Verification items for the finished model (mm, model axes). Face numbers are marked on the shaded views. A direction names the side the tool comes from. Coordinates: 2 decimals unless noted, no trailing zeros. Order: outer loops, then holes, each group sorted by start corner. A loop starts at its lowest first (then second) coordinate and runs counter-clockwise, first axis right, second up.
Q1. Cross-section at A-A, the plane y = 0. Count the separate pieces of the cut face and the enclosed holes in it, and give its area (3 significant figures).
Q2. Set-up check for the marked faces 4 and 5: record each of +Z, -Z, +X, -X, +Y, -Y from which the full face is reachable in a straight line by a thin tool's end or side.
Q3. Thickness scan on line 1 (Y direction, x = -39.5, z = -2); line 2 (X direction, y = 7.5, z = -2.25); line 3 (X direction, y = -6, z = -6). Record the ranges inside material, lowest first.
Q4. Depth check by flat-ended pin: P1, Ø5, axis at x = 1.5, z = -4.5, coming from the +Y side; P2, Ø5, axis at x = -24.18, y = 0, coming from the +Z side; P3, Ø2, axis at x = -18.5, z = -4, coming from the +Y side; P4, Ø3, axis at y = 3.5, z = -6, coming from the +X side. Enter the tip coordinate at first touch or a pass-through.
Q5. Draft check along X on the marked faces 1, 2 and 3. Enter one of: pulls with the +X half, pulls with the -X half, needs draft (parallel to the pull), parting line crosses it, or undercut.
Q6. Cross-section at D-D, the plane x = 55. Record the boundary of the cut face in (y, z).
Q7. Cross-section at B-B, the plane y = 33. Record the boundary of the cut face in (x, z).
from build123d import *

# Parameters (mm, degrees)
SKETCH6_R                        = 29
SKETCH6_R_2                      = 20
INNER_RING_DEPTH                 = 10
MOTOR_CONNECTOR_CUT_DEPTH        = 10
SKETCH8_R                        = 2.25
MOTOR_CONNECTOR_HOLES_DEPTH      = 1
MOTOR_CONNECTOR_HOLES_DEPTH_BACK = 18
MIDDLE_PATTERN_DEPTH             = 10
SKETCH9_R                        = 60
SKETCH9_R_2                      = 50
SKETCH9_R_3                      = 2.5
BOSS_EXTRUDE1_DEPTH              = 10


with BuildPart() as part:
    # Sketch6 → Inner Ring (new body)
    with BuildSketch(Plane.XY):
        Circle(SKETCH6_R)
        Circle(SKETCH6_R_2, mode=Mode.SUBTRACT)
    extrude(amount=-INNER_RING_DEPTH)

    # Sketch7 → Motor Connector Cut (add)
    with BuildSketch(Plane.XY):
        with BuildLine():
            ThreePointArc((20, 0), (19.840593925, 2.52008585), (19.364916731, 5))
            Line((19.364916731, 5), (9.999996731, 5))
            Line((9.999996731, 5), (9.999996731, -5))
            Line((9.999996731, -5), (19.364916731, -5))
            ThreePointArc((19.364916731, -5), (19.840593925, -2.52008585), (20, 0))
        make_face()
        with BuildLine():
            ThreePointArc((5, 19.364916731), (0, 20), (-5, 19.364916731))
            Line((-5, 19.364916731), (-5, 9.999996731))
            Line((-5, 9.999996731), (5, 9.999996731))
            Line((5, 9.999996731), (5, 19.364916731))
        make_face()
        with BuildLine():
            Line((-9.999996731, -5), (-9.999996731, 5))
            Line((-9.999996731, 5), (-19.364916731, 5))
            ThreePointArc((-19.364916731, 5), (-20, 0), (-19.364916731, -5))
            Line((-19.364916731, -5), (-9.999996731, -5))
        make_face()
        with BuildLine():
            Line((-5, -9.999996731), (-5, -19.364916731))
            ThreePointArc((-5, -19.364916731), (0, -20), (5, -19.364916731))
            Line((5, -19.364916731), (5, -9.999996731))
            Line((5, -9.999996731), (-5, -9.999996731))
        make_face()
    extrude(amount=-MOTOR_CONNECTOR_CUT_DEPTH)

    # Sketch8 → Motor Connector Holes (cut, two sides)
    with BuildSketch(Plane.XY) as motor_connector_holes_sk:
        with Locations((0, 24.182458366)):
            Circle(SKETCH8_R)
        with Locations((24.182458366, 0)):
            Circle(SKETCH8_R)
        with Locations((0, -24.182458366)):
            Circle(SKETCH8_R)
        with Locations((-24.182458366, 0)):
            Circle(SKETCH8_R)
    extrude(amount=MOTOR_CONNECTOR_HOLES_DEPTH, mode=Mode.SUBTRACT)
    extrude(motor_connector_holes_sk.sketch, amount=-MOTOR_CONNECTOR_HOLES_DEPTH_BACK, mode=Mode.SUBTRACT)

    # Sketch10 → Middle Pattern (add)
    with BuildSketch(Plane.XY):
        with BuildLine():
            ThreePointArc((28.607215414, 4.756808408), (26.539406056, -11.690163651), (15.800414568, -24.317625284))
            ThreePointArc((15.800414568, -24.317625284), (10.393277118, -43.149392299), (-8.201394307, -49.322785114))
            ThreePointArc((-8.201394307, -49.322785114), (15.267827816, -47.611904328), (35.355339059, -35.355339059))
            ThreePointArc((35.355339059, -35.355339059), (42.321804958, -13.559663633), (28.607215414, 4.756808408))
        make_face()
        with BuildLine():
            ThreePointArc((24.317625284, 15.800414568), (43.149392359, 10.39327706), (49.322785087, -8.201394473))
            ThreePointArc((49.322785087, -8.201394473), (47.611904354, 15.267827736), (35.355339059, 35.355339059))
            ThreePointArc((35.355339059, 35.355339059), (13.559663633, 42.321804958), (-4.756808408, 28.607215414))
            ThreePointArc((-4.756808408, 28.607215414), (11.690163651, 26.539406056), (24.317625284, 15.800414568))
        make_face()
        with BuildLine():
            ThreePointArc((8.201394106, 49.322785148), (-15.267827902, 47.611904301), (-35.355339044, 35.355339075))
            ThreePointArc((-35.355339044, 35.355339075), (-42.32180496, 13.559663644), (-28.607215414, -4.756808408))
            ThreePointArc((-28.607215414, -4.756808408), (-26.539406056, 11.690163651), (-15.800414568, 24.317625284))
            ThreePointArc((-15.800414568, 24.317625284), (-10.393277189, 43.149392225), (8.201394106, 49.322785148))
        make_face()
        with BuildLine():
            ThreePointArc((4.756808408, -28.607215414), (-11.690163651, -26.539406056), (-24.317625284, -15.800414568))
            ThreePointArc((-24.317625284, -15.800414568), (-43.149392012, -10.393277393), (-49.322785244, 8.201393524))
            ThreePointArc((-49.322785244, 8.201393524), (-47.61190416, -15.267828343), (-35.355338839, -35.35533928))
            ThreePointArc((-35.355338839, -35.35533928), (-13.559663479, -42.321804932), (4.756808408, -28.607215414))
        make_face()
    extrude(amount=-MIDDLE_PATTERN_DEPTH)

    # Sketch9 → Boss-Extrude1 (add)
    with BuildSketch(Plane.XY):
        Circle(SKETCH9_R)
        Circle(SKETCH9_R_2, mode=Mode.SUBTRACT)
        with Locations((0, 55)):
            Circle(SKETCH9_R_3, mode=Mode.SUBTRACT)
        with Locations((-38.890872965, 38.890872965)):
            Circle(SKETCH9_R_3, mode=Mode.SUBTRACT)
        with Locations((-55, 0)):
            Circle(SKETCH9_R_3, mode=Mode.SUBTRACT)
        with Locations((-38.890872965, -38.890872965)):
            Circle(SKETCH9_R_3, mode=Mode.SUBTRACT)
        with Locations((0, -55)):
            Circle(SKETCH9_R_3, mode=Mode.SUBTRACT)
        with Locations((38.890872965, -38.890872965)):
            Circle(SKETCH9_R_3, mode=Mode.SUBTRACT)
        with Locations((55, 0)):
            Circle(SKETCH9_R_3, mode=Mode.SUBTRACT)
        with Locations((38.890872965, 38.890872965)):
            Circle(SKETCH9_R_3, mode=Mode.SUBTRACT)
    extrude(amount=-BOSS_EXTRUDE1_DEPTH)


solid = part.part
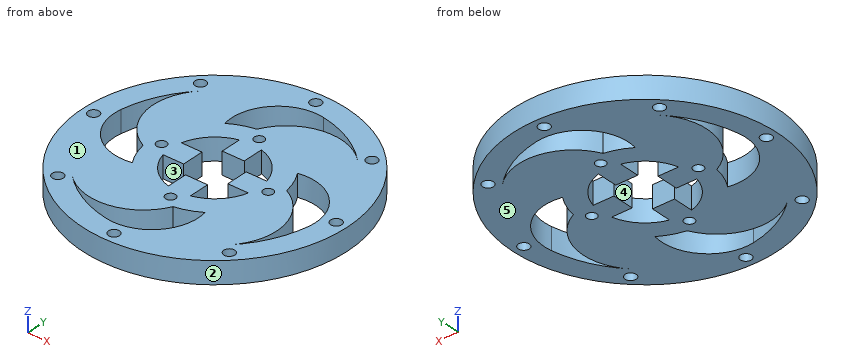
Check values:
1. separate pieces: 8
1. enclosed holes: 0
1. area: 535 mm2
2. face 4: +Z, -Z
2. face 5: -Z, +X, -X, +Y, -Y
3. line 1: y = -45.16 to -41.32, -36.47 to -13.2, 5.53 to 29.87, 30.66 to 36.47, 41.32 to 45.16
3. line 2: x = -59.53 to -49.43, -40.49 to -18.54, 18.54 to 28.01, 45.66 to 59.53
3. line 3: x = -59.7 to -46.64, -28.37 to -19.08, 19.08 to 39.76, 49.57 to 59.7
4. P1: stops at y = 60
4. P2: stops at z = 0
4. P3: stops at y = 57.39
4. P4: stops at x = 59.97
5. face 1: needs draft
5. face 2: parting line crosses it
5. face 3: undercut
6. outline: (-23.98, -10) - (-2.5, -10) - (-2.5, 0) - (-23.98, 0) - close; (2.5, -10) - (23.98, -10) - (23.98, 0) - (2.5, 0) - close
7. outline: (-50.11, -10) - (-37.56, -10) - (-37.56, 0) - (-50.11, 0) - close; (-37.43, -10) - (-15.78, -10) - (-15.78, 0) - (-37.43, 0) - close; (-2.03, -10) - (50.11, -10) - (50.11, 0) - (-2.03, 0) - close
